Autodesk Inventor part; units mm, degrees
ref_plane "YZ Plane" through (0, 0, 0) normal (1, 0, 0) x (0, 1, 0)
ref_plane "XZ Plane" through (0, 0, 0) normal (0, 1, 0) x (-1, 0, 0)
ref_plane "XY Plane" through (0, 0, 0) normal (0, 0, 1) x (1, 0, 0)
sketch "Sketch1" plane through (0, 0, 0) normal (0, 1, 0) x (-1, 0, 0)
  line L0 (-304.8, 101.6) -> (304.8, 101.6)
  line L1 (304.8, 101.6) -> (304.8, -101.6)
  line L2 (304.8, -101.6) -> (-304.8, -101.6)
  line L3 (-304.8, -101.6) -> (-304.8, 101.6)
  line L4 (-304.8, 101.6) -> (304.8, -101.6) construction
  line L5 (304.8, 101.6) -> (-304.8, -101.6) construction
  point P0 (0, 0)
  dimension "length" = 609.6
  dimension "width" = 203.2
extrude "Extrusion1" add sketch "Sketch1" along normal blind 19.05
sketch "Sketch2" plane through (0, 19.05, 0) normal (0, 1, 0) x (1, 0, 0)
  line L0 (-304.8, -101.6) -> (304.8, -101.6)
  line L1 (304.8, 101.6) -> (-304.8, 101.6)
  line L2 (-304.8, -101.6) -> (-304.8, 101.6)
  line L3 (-304.8, 101.6) -> (-285.75, 101.6)
  line L4 (-285.75, 101.6) -> (-285.75, -101.6)
  line L5 (-285.75, -101.6) -> (-304.8, -101.6)
  point P0 (0, 0)
  dimension "d4" = 19.05
extrude "Extrusion2" add sketch "Sketch2" along normal blind 190.5
mirror "Mirror2" about plane through (0, 0, 0) normal (1, 0, 0) of "Extrusion2"
sketch "Sketch3" plane through (0, 19.05, 0) normal (0, 1, 0) x (1, 0, 0)
  line L0 (-285.75, -101.6) -> (-247.65, -101.6)
  line L1 (-247.65, -101.6) -> (-247.65, -82.55)
  line L2 (-247.65, -82.55) -> (-285.75, -82.55)
  line L3 (-285.75, -82.55) -> (-285.75, -101.6)
  line L4 (-285.75, -101.6) -> (285.75, -101.6)
  line L5 (285.75, -101.6) -> (247.65, -101.6)
  line L6 (247.65, -101.6) -> (247.65, -82.55)
  line L7 (247.65, -82.55) -> (285.75, -82.55)
  line L8 (285.75, -82.55) -> (285.75, -101.6)
  point P0 (0, 0)
  dimension "d7" = 19.05
  dimension "d8" = 19.05
  dimension "d12" = 38.1
  dimension "d14" = 38.1
extrude "Extrusion3" add sketch "Sketch3" along normal blind 25.4
mirror "Mirror3" about plane through (0, 0, 0) normal (0, 0, 1) of "Extrusion3"
sketch "Sketch5" plane through (0, 209.55, 0) normal (0, 1, 0) x (1, 0, 0)
  line L0 (304.8, -101.6) -> (-304.8, -101.6)
  line L1 (304.8, 101.6) -> (304.8, -101.6)
  line L2 (-304.8, -101.6) -> (304.8, -101.6)
  line L3 (304.8, -101.6) -> (304.8, 101.6)
  line L4 (304.8, 101.6) -> (-304.8, 101.6)
  line L5 (-304.8, 101.6) -> (-304.8, -101.6)
  point P0 (0, 0)
extrude "Extrusion4" add sketch "Sketch5" along normal blind 19.05
equation "\"d4\" = thickness"
equation "\"d7\" = thickness"
equation "\"d8\" = thickness"
equation "\"d14\" = d12"
equation "\"d15\" = thickness"
properties part number "cabinet" material "Pine, Radiata"
Geometry check sheet. Reference: the model listing, model coordinates, mm. A direction names the side the tool comes from. Give positions to 0.01 mm unless a question says otherwise; leave off trailing zeros. Order: outer loops, then holes, each group sorted by start corner. A loop starts at its lowest first (then second) coordinate and runs counter-clockwise, first axis right, second up. Notation, with made-up numbers: (28, 22) - (72, 22) arc R30 ccw to (72, 56) - close; hole circle Ø4 at (22, 21). An arc over 180 degrees is marked (long way). Write item = value, one per line. Start each with the question number.
1) Section check B-B (y = 174.5). Enter the section's corners in (x, z).
2) Section check C-C (z = 14). Enter the section's corners in (x, y).
3) Access from +Z, -Z, +X, -X, +Y, -Y to the whole of each face (thin tool, end or side, straight path). Record for faces 1 (the flat face through (4, 0, 1)), 2 (the flat face through (4, 19.05, 1)), 3 (the flat face through (247.65, 32, 92)).
4) Scan lines: L1, parallel to Y at x = -61.5, z = -1; L2, parallel to X at y = 196, z = 40. Record each from-to range of solid material in increasing order.
5) Section check A-A (x = 264). Enter the section's corners in (y, z).
6) Draft check along Z on faces 4 (the flat face through (266, 32, 82.55)), 5 (the flat face through (1, 12, 101.6)), 6 (the flat face through (-247.65, 32, 92)). Enter one of: released by +Z, released by -Z, zero draft, split by the parting line, or undercut.
7) Section check D-D (x = -99.5). Enter the section's corners in (y, z), then the cut area to 3 significant figures.
Geometry check:
q1.outline = (-304.8, -101.6) - (-285.75, -101.6) - (-285.75, 101.6) - (-304.8, 101.6) - close; (285.75, -101.6) - (304.8, -101.6) - (304.8, 101.6) - (285.75, 101.6) - close
q2.outline = (-304.8, 0) - (304.8, 0) - (304.8, 228.6) - (-304.8, 228.6) - close; hole (-285.75, 19.05) - (285.75, 19.05) - (285.75, 209.55) - (-285.75, 209.55) - close
q3.face_1 = +Z, -Z, +X, -X, -Y
q3.face_2 = none
q3.face_3 = +Z, -Z
q4.L1 = 0 to 19.05, 209.55 to 228.6
q4.L2 = -304.8 to -285.75, 285.75 to 304.8
q5.outline = (0, -101.6) - (44.45, -101.6) - (44.45, -82.55) - (19.05, -82.55) - (19.05, 82.55) - (44.45, 82.55) - (44.45, 101.6) - (0, 101.6) - close; (209.55, -101.6) - (228.6, -101.6) - (228.6, 101.6) - (209.55, 101.6) - close
q6.face_4 = undercut
q6.face_5 = released by +Z
q6.face_6 = zero draft
q7.outline = (0, -101.6) - (19.05, -101.6) - (19.05, 101.6) - (0, 101.6) - close; (209.55, -101.6) - (228.6, -101.6) - (228.6, 101.6) - (209.55, 101.6) - close
q7.area = 7,740 mm2
